Could you check a few things on this model? Use its own coordinates, in mm. Face numbers are marked on the shaded views. A direction names the side the tool comes from. Round coordinates to 2 decimals unless told otherwise and drop trailing zeros. Write each loop counter-clockwise with the first axis right and the second up, starting at its lowest first coordinate (ties: lowest second). Pieces come first, ordered by that corner, then holes. Notation, with made-up numbers: (-17.5, 44) -> (-5.5, 44) arc R13 ccw to (-5.5, 60) -> close; hole circle Ø5 at (56, 68.5). An arc over 180 degrees is marked (long way). Answer as CSV lines item,"result". Start each with the question number.
Q1. For the marked faces 1, 2, 3 and 4, which set-ups out of +Z, -Z, +X, -X, +Y, -Y let a thin tool reach every point of the face, with its end or its side?
Q2. Imagine slicing it at A-A on x = 8.75. Please give me the cut outline in (y, z), and give its area (3 significant figures).
Q3. Will these pins go through, and if not, where does the flat tip stop? pin 1 Ø0.8 at (y, z) = (-12.5, 1.5) entering from -X; pin 2 Ø0.5 at (y, z) = (-9, 2) entering from -X; pin 3 Ø1.1 at (x, z) = (-9.5, 2) entering from -Y.
Q4. Imagine slicing it at B-B on y = 10.75. Please give me the cut outline in (x, z), and give its area (3 significant figures).
Q5. If I drill on line 1 (Y direction, x = 2.25, z = 0.75); line 2 (Y direction, x = 9.5, z = 2.2); line 3 (X direction, y = -5.5, z = 3.05), over which ranges is the centre line in solid material (lowest first)? Write a range as [from, to].
Q6. Imagine slicing it at C-C on x = -10.75. Please give me the cut outline in (y, z), and give its area (3 significant figures).
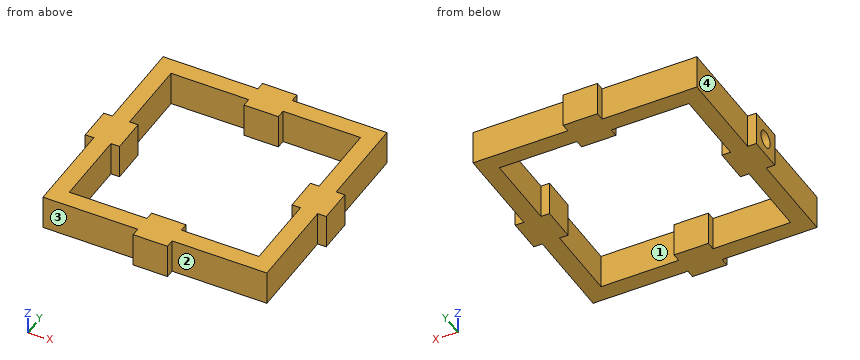
from build123d import *

# Parameters (mm, degrees)
BOSS_EXTRUDE1_DEPTH = 4
SKETCH3_R           = 1
CUT_EXTRUDE1_DEPTH  = 3


with BuildPart() as part:
    # Sketch1 → Boss-Extrude1 (new body)
    with BuildSketch(Plane.XY):
        Polygon((-12.961370769, -0.721570782), (-11.961370769, -0.721570782), (-11.961370769, -11.721570782), (-4.331288589, -11.721570782), (-0.917373368, -11.721570782), (-0.917373368, -12.721570782), (3.082626632, -12.721570782), (3.082626632, -11.721570782), (14.126624033, -11.721570782), (14.126624033, -0.721570782), (15.126624033, -0.721570782), (15.126624033, 3.278429218), (14.126624033, 3.278429218), (14.126624033, 14.278429218), (3.082626632, 14.278429218), (3.082626632, 15.278429218), (-0.917373368, 15.278429218), (-0.917373368, 14.278429218), (-11.961370769, 14.278429218), (-11.961370769, 3.278429218), (-12.961370769, 3.278429218), align=None)
        Polygon((3.082626632, 12.278429218), (12.126624033, 12.278429218), (12.126624033, 3.278429218), (11.126624033, 3.278429218), (11.126624033, -0.721570782), (12.126624033, -0.721570782), (12.126624033, -9.721570782), (3.082626632, -9.721570782), (3.082626632, -8.721570782), (-0.917373368, -8.721570782), (-0.917373368, -9.721570782), (-4.331288589, -9.721570782), (-9.961370769, -9.721570782), (-9.961370769, -0.721570782), (-8.961370769, -0.721570782), (-8.961370769, 3.278429218), (-9.961370769, 3.278429218), (-9.961370769, 12.278429218), (-0.917373368, 12.278429218), (-0.917373368, 11.278429218), (3.082626632, 11.278429218), align=None, mode=Mode.SUBTRACT)
    extrude(amount=BOSS_EXTRUDE1_DEPTH)

    # Sketch3 → Cut-Extrude1 (cut)
    with BuildSketch(Plane.ZY.offset(12.961370769)):
        with Locations(Location((2, 1.278429218, 0), (0, 0, 270))):
            Circle(SKETCH3_R)
    extrude(amount=-CUT_EXTRUDE1_DEPTH, mode=Mode.SUBTRACT)


solid = part.part
Checks:
1,face 1,"+Z, -Z"
1,face 2,"+Z, -Z, +X, -Y"
1,face 3,"+Z, -Z, -X, -Y"
1,face 4,"+Z, -Z, -X, +Y"
2,outline,"(-11.72, 0) -> (-9.72, 0) -> (-9.72, 4) -> (-11.72, 4) -> close; (12.28, 0) -> (14.28, 0) -> (14.28, 4) -> (12.28, 4) -> close"
2,area,"16.0 mm^2"
3,pin 1,"x = -0.92"
3,pin 2,"x = -11.96"
3,pin 3,"y = -11.72"
4,outline,"(-11.96, 0) -> (-9.96, 0) -> (-9.96, 4) -> (-11.96, 4) -> close; (12.13, 0) -> (14.13, 0) -> (14.13, 4) -> (12.13, 4) -> close"
4,area,"16.0 mm^2"
5,line 1,"[-12.72, -8.72], [11.28, 15.28]"
5,line 2,"[-11.72, -9.72], [12.28, 14.28]"
5,line 3,"[-11.96, -9.96], [12.13, 14.13]"
6,outline,"(-11.72, 0) -> (14.28, 0) -> (14.28, 4) -> (-11.72, 4) -> close; hole circle Ø2 at (1.28, 2)"
6,area,"101 mm^2"
